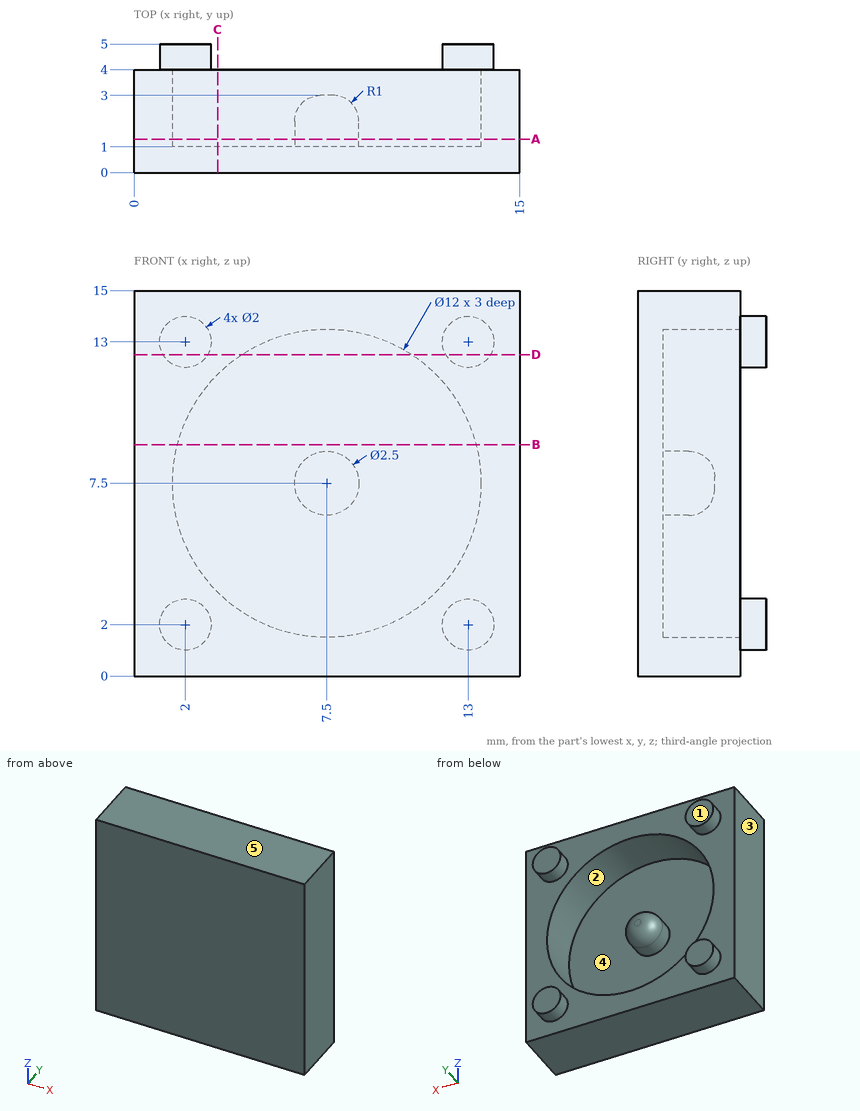
Geometry: see drawing. Coordinates: mm, zero at the bounding-box minimum. A direction names the side the tool comes from. Coordinates: 2 decimals unless noted, no trailing zeros. Loops run counter-clockwise (first coordinate to the right, second up) from the corner with the lowest first, then second, coordinate; pieces in that order, holes last.
(1) Pull-direction query (X, two-part tool) for the marked faces 1, 2 and 3; classes: released by +X, released by -X, zero draft, split by the parting line, or undercut.
(2) Set-up query: the marked faces 4 and 5. Return all of +Z, -Z, +X, -X, +Y, -Y with unobstructed straight access to the full face (end or side cutting, diameter ignored); none if empty.
(3) Section B-B on z = 9. Return the cut outline in (x, y).
(4) First-contact query: pin 1 Ø5 at (x, z) = (11.5, 10.5) entering from +Y; pin 2 Ø4.5 at (x, z) = (10.5, 8.5) entering from +Y. Flat tips, straight axial feed; report the tip coordinate or a pass-through.
(5) Section A-A on y = 1.3. Return the cut outline in (x, z).
(6) Material intervals for probe 1 along X at (y, z) = (1.7, 7.5); probe 2 along Z at (x, y) = (7.5, 3.2), sorted ascending.
(7) Section C-C on x = 3.25. Return the cut outline in (y, z).
(8) Section D-D on z = 12.5. Return the cut outline in (x, y), then the cut area to 3 significant figures.
Data:
1. face 1: zero draft
1. face 2: undercut
1. face 3: released by -X
2. face 4: +Y
2. face 5: +Z, +X, -X, +Y, -Y
3. outline: (0, 0) - (15, 0) - (15, 4) - (13.31, 4) - (13.31, 1) - (1.69, 1) - (1.69, 4) - (0, 4) - close
4. pin 1: stops at y = 5
4. pin 2: stops at y = 2.75
5. outline: (0, 0) - (15, 0) - (15, 15) - (0, 15) - close; circle Ø2.5 at (7.5, 7.5); hole circle Ø12 at (7.5, 7.5)
6. probe 1: x = 0 to 1.5, 6.25 to 8.75, 13.5 to 15
6. probe 2: z = 0 to 1.5, 13.5 to 15
7. outline: (0, 0) - (4, 0) - (4, 3.26) - (1, 3.26) - (1, 11.74) - (4, 11.74) - (4, 15) - (0, 15) - close
8. outline: (0, 0) - (15, 0) - (15, 4) - (13.87, 4) - (13.87, 5) - (12.13, 5) - (12.13, 4) - (10.82, 4) - (10.82, 1) - (4.18, 1) - (4.18, 4) - (2.87, 4) - (2.87, 5) - (1.13, 5) - (1.13, 4) - (0, 4) - close
8. area: 43.6 mm2
